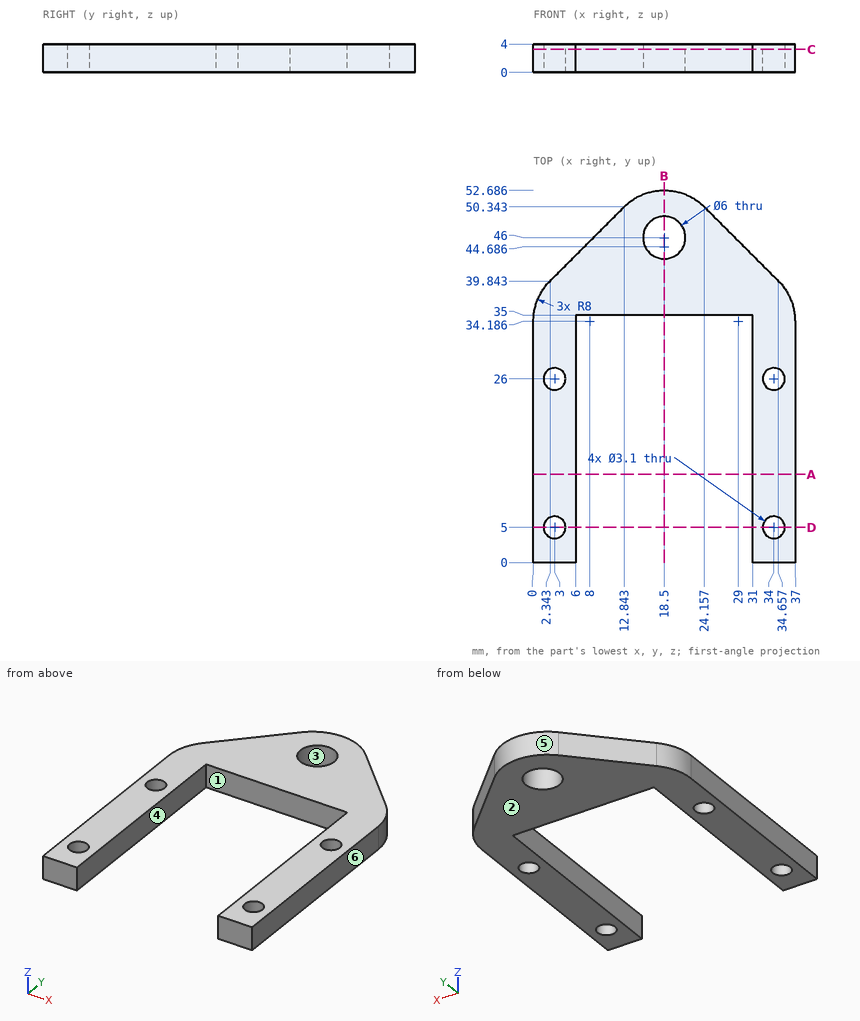
Input: dimensioned drawing with shaded views. Units: mm. Origin: part minimum x, y, z. A direction names the side the tool comes from. Give positions to 0.01 mm unless a question says otherwise; leave off trailing zeros. Write each loop counter-clockwise with the first axis right and the second up, starting at its lowest first coordinate (ties: lowest second). Pieces come first, ordered by that corner, then holes.
1. Section query A-A, the plane y = 12.5. Return loops of the section in (x, z), then the cut area to 3 significant figures.
2. Reachability of the marked faces 1 and 2 from +Z, -Z, +X, -X, +Y, -Y: full face, straight path, thin tool, end or side. Return the list, or none.
3. Pin query (flat end, axial travel): P1, Ø3, axis at x = 3, y = 5, coming from the +Z side; P2, Ø2, axis at x = 12, z = 3, coming from the -Y side. Return the tip coordinate at first contact, or that it passes through.
4. Section query D-D, the plane y = 5. Return loops of the section in (x, z).
5. Section query B-B, the plane x = 18.5. Return loops of the section in (y, z).
6. Line query: probe 1 along X at (y, z) = (18.5, 2.95); probe 2 along Y at (x, z) = (3, 1.4); probe 3 along Y at (x, z) = (16, 1.5) (1 decimal). Output: solid intervals per line, ascending.
7. Section query C-C, the plane z = 3.25. Return loops of the section in (x, y).
8. Draft query along X for the marked faces 3, 4, 5 and 6. Return one class per face: released by +X, released by -X, zero draft, split by the parting line, or undercut.
Computed:
1. outline: (0, 0) - (6, 0) - (6, 4) - (0, 4) - close; (31, 0) - (37, 0) - (37, 4) - (31, 4) - close
1. area: 48.0 mm2
2. face 1: +Z, -Z, -Y
2. face 2: -Z, +X, -X, +Y, -Y
3. P1: passes through
3. P2: stops at y = 35
4. outline: (0, 0) - (1.45, 0) - (1.45, 4) - (0, 4) - close; (4.55, 0) - (6, 0) - (6, 4) - (4.55, 4) - close; (31, 0) - (32.45, 0) - (32.45, 4) - (31, 4) - close; (35.55, 0) - (37, 0) - (37, 4) - (35.55, 4) - close
5. outline: (35, 0) - (43, 0) - (43, 4) - (35, 4) - close; (49, 0) - (52.69, 0) - (52.69, 4) - (49, 4) - close
6. probe 1: x = 0 to 6, 31 to 37
6. probe 2: y = 0 to 3.45, 6.55 to 24.45, 27.55 to 40.5
6. probe 3: y = 35 to 44.3, 47.7 to 52.3
7. outline: (0, 0) - (6, 0) - (6, 35) - (31, 35) - (31, 0) - (37, 0) - (37, 34.19) arc R8 ccw to (34.66, 39.84) - (24.16, 50.34) arc R8 ccw to (12.84, 50.34) - (2.34, 39.84) arc R8 ccw to (0, 34.19) - close; hole circle Ø3.1 at (3, 5); hole circle Ø3.1 at (3, 26); hole circle Ø6 at (18.5, 46); hole circle Ø3.1 at (34, 5); hole circle Ø3.1 at (34, 26)
8. face 3: undercut
8. face 4: undercut
8. face 5: split by the parting line
8. face 6: released by +X
